```python
from build123d import *

# Parameters (mm, degrees)
SKETCH_R             = 47.5
SKETCH_R_2           = 6
PAD_DEPTH            = 5
SKETCH001_R          = 6
PAD001_DEPTH         = 20
FILLET_R             = 30
POCKET_DEPTH         = 1
SKETCH003_R          = 2.75
POCKET001_DEPTH      = 320.814007
POCKET001_DEPTH_BACK = 320.814007
POLARPATTERN_COUNT   = 3
FILLET001_R          = 5


with BuildPart() as part:
    # Sketch → Pad (new body)
    with BuildSketch(Plane.XY):
        Circle(SKETCH_R)
        Circle(SKETCH_R_2, mode=Mode.SUBTRACT)
    extrude(amount=PAD_DEPTH)

    # Sketch001 → Pad001 (join)
    with BuildSketch(Plane.XY):
        Polygon((16, 9.237604), (16, 40), (11, 40), (11, 10), (-11, 10), (-11, 40), (-16, 40), (-16, 9.237604), (-42.641016, -6.143594), (-40.141016, -10.473721), (-14.160254, 4.526279), (-3.160254, -14.526279), (-29.141016, -29.526279), (-26.641016, -33.856406), (0, -18.475209), (26.641016, -33.856406), (29.141016, -29.526279), (3.160254, -14.526279), (14.160254, 4.526279), (40.141016, -10.473721), (42.641016, -6.143594), align=None)
        Circle(SKETCH001_R, mode=Mode.SUBTRACT)
    extrude(amount=-PAD001_DEPTH)

    # Fillet
    fillet_edges = [part.edges().sort_by_distance(p)[0] for p in [
        (16, 9.237604, -10),
        (-16, 9.237604, -10),
        (0, -18.475209, -10),
    ]]
    fillet(fillet_edges, radius=FILLET_R)

    # Sketch002 (on Face14 of Fillet) → Pocket (cut)
    with BuildSketch(Plane(origin=(-16, 0, 0), x_dir=(0, -1, 0), z_dir=(-1, 0, 0))):
        Polygon((-28, -12.309401), (-28, -7.690599), (-32, -5.381198), (-36, -7.690599), (-36, -12.309401), (-32, -14.618802), align=None)
    pocket = extrude(amount=-POCKET_DEPTH, mode=Mode.SUBTRACT)

    # Sketch003 → Pocket001 (cut, two sides)
    with BuildSketch(Plane.YZ) as pocket001_sk:
        with Locations((32, -10)):
            Circle(SKETCH003_R)
    pocket001 = extrude(amount=-POCKET001_DEPTH, mode=Mode.SUBTRACT) + extrude(pocket001_sk.sketch, amount=POCKET001_DEPTH_BACK, mode=Mode.SUBTRACT)

    # PolarPattern: Pocket, Pocket001 ×3 about axis
    polarpattern_axis = Axis((0, 0, 0), (0, 0, 1))
    for i in range(1, POLARPATTERN_COUNT):
        add(pocket.rotate(polarpattern_axis, i * 360 / POLARPATTERN_COUNT), mode=Mode.SUBTRACT)
        add(pocket001.rotate(polarpattern_axis, i * 360 / POLARPATTERN_COUNT), mode=Mode.SUBTRACT)

    # Fillet001
    fillet001_edges = [part.edges().sort_by_distance(p)[0] for p in [
        (14.160254, 4.526279, -10),
        (3.160254, -14.526279, -10),
        (11, 10, -10),
        (-11, 10, -10),
        (-14.160254, 4.526279, -10),
        (-3.160254, -14.526279, -10),
        (-8.660254, -5, 0),
        (0, 10, 0),
        (8.660254, -5, 0),
        (20.019238, 11.558112, 0),
        (-20.019238, 11.558112, 0),
        (0, -23.116225, 0),
    ]]
    fillet(fillet001_edges, radius=FILLET001_R)


solid = part.part
```
CAD build for the part. Positions are in the model's coordinates, mm. A direction names the side the tool comes from. Coordinates: 2 decimals unless noted, no trailing zeros. Write each loop counter-clockwise with the first axis right and the second up, starting at its lowest first coordinate (ties: lowest second). Pieces come first, ordered by that corner, then holes.
(1) Cut at C-C, the plane z = -10. Count the separate pieces of the cut face and the enclosed holes in it, and give its area (3 significant figures).
(2) Drill centre lines: probe 1 along Z at (x, y) = (13.05, 32); probe 2 along Y at (x, z) = (13.35, -10); probe 3 along Z at (x, y) = (11, -42.5). Where is each one in solid material? Low to high.
(3) 3-axis set-ups, long thin cutter, end or side, ignore diameter. For faces 1 (the face through (-21.667, -30.415, -6.52)), 2 (the face through (-15.51, 33.97, -6.52)), 3 (the face through (41.495, -8.129, -9.86)): which of +Z, -Z, +X, -X, +Y, -Y reach the whole face in a straight line?
(4) Two-plate mould, pull along Y, no slides. Class faces 4 (the face through (16, 35, -12)), 5 (the face through (-15.51, 30.03, -13.48)), 6 (the face through (-41.565, -8.007, -9.86)): +Y half, -Y half, draft (parallel to the pull), parting line (faces both ways), or undercut.
(5) Cut at B-B, the plane y = 30.5. List the corners of the cut face in (x, z), and give its area (3 significant figures).
(6) Flat gauge pins, fed straight in: pin 1 (2 mm diameter, centred on y = -36.5, z = -3.5, fed in from +X); pin 2 (4 mm diameter, centred on y = -0.5, z = -13, fed in from -X); pin 3 (4 mm diameter, centred on y = 36, z = -10, fed in from +X); pin 4 (1.5 mm diameter, centred on x = -26, y = 10, fed in from -Z). Where does each tip first touch, or does it go through?
Geometry says:
1. separate pieces: 7
1. enclosed holes: 1
1. area: 1,310 mm2
2. probe 1: z = -20 to -12.75, -7.25 to 5
2. probe 2: y = -26.25 to -20.41, 1.94 to 29.25, 34.75 to 40
2. probe 3: z = 0 to 5
3. face 1: none
3. face 2: -X
3. face 3: -Z, +X, -Y
4. face 4: draft
4. face 5: undercut
4. face 6: -Y half
5. outline: (-36.41, 0) - (-21, 0) arc R5 cw to (-16, -5) - (-16, -6.25) - (-15, -6.25) - (-15, -7.7) - (-11, -7.7) - (-11, 0) - (11, 0) - (11, -7.7) - (16, -7.7) - (16, -5) arc R5 cw to (21, 0) - (36.41, 0) - (36.41, 5) - (-36.41, 5) - close; (-16, -20) - (-11, -20) - (-11, -12.3) - (-15, -12.3) - (-15, -13.75) - (-16, -13.75) - close; (11, -20) - (16, -20) - (16, -12.3) - (11, -12.3) - close
5. area: 526 mm2
6. pin 1: passes through
6. pin 2: stops at x = -36.33
6. pin 3: stops at x = 16
6. pin 4: stops at z = -0.3
